CAD build for the part. Positions are in the model's coordinates, mm. Round coordinates to 2 decimals unless told otherwise and drop trailing zeros. Write each loop counter-clockwise with the first axis right and the second up, starting at its lowest first coordinate (ties: lowest second). Pieces come first, ordered by that corner, then holes. Notation, with made-up numbers: (49, 57.5) - (57, 57.5) arc R10 ccw to (57, 61.5) - close; hole circle Ø9 at (21.25, -9). An arc over 180 degrees is marked (long way). Answer in a Markdown table with one row per item.
```python
from build123d import *

# Parameters (mm, degrees)
SKETCH4_R           = 42.545
BOSS_EXTRUDE2_DEPTH = 0.254
SKETCH5_R           = 29.845
CUT_EXTRUDE5_DEPTH  = 1.254
SKETCH6_R           = 4.699
CUT_EXTRUDE6_DEPTH  = 1.254
SKETCH8_OUTSIDE_W   = 111.158
SKETCH8_OUTSIDE_H   = 111.158
CUT_EXTRUDE11_DEPTH = 1.254


with BuildPart() as part:
    # Sketch4 → Boss-Extrude2 (new body)
    with BuildSketch(Plane.XY):
        Circle(SKETCH4_R)
    extrude(amount=BOSS_EXTRUDE2_DEPTH)

    # Sketch5 → Cut-Extrude5 (cut, through all)
    with BuildSketch(Plane.XY.offset(0.254)):
        Circle(SKETCH5_R)
    extrude(amount=-CUT_EXTRUDE5_DEPTH, mode=Mode.SUBTRACT)

    # Sketch6 → Cut-Extrude6 (cut, through all)
    with BuildSketch(Plane.XY.offset(0.254)):
        with Locations((36.195, 0)):
            Circle(SKETCH6_R)
    extrude(amount=-CUT_EXTRUDE6_DEPTH, mode=Mode.SUBTRACT)

    # Sketch8 outside → Cut-Extrude11 (cut, through all)
    with BuildSketch(Plane.XY.offset(0.254)):
        Rectangle(SKETCH8_OUTSIDE_W, SKETCH8_OUTSIDE_H)
        with BuildLine():
            Line((28.034216891, -10.237514752), (39.774946424, -15.100684157))
            ThreePointArc((39.774946424, -15.100684157), (42.545, 0), (39.774946424, 15.100684157))
            Line((39.774946424, 15.100684157), (28.034216891, 10.237514752))
            ThreePointArc((28.034216891, 10.237514752), (29.845, 0), (28.034216891, -10.237514752))
        make_face(mode=Mode.SUBTRACT)
    extrude(amount=-CUT_EXTRUDE11_DEPTH, mode=Mode.SUBTRACT)


solid = part.part
```
Q1. Saw through at B-B on z = 0.1. List the corners of the cut face in (x, y) (3 decimals).
Computed:
| item | result |
|---|---|
| outline | (28.034, -10.238) - (39.775, -15.101) arc R42.545 ccw to (39.775, 15.101) - (28.034, 10.238) arc R29.845 cw to start; hole circle Ø9.398 at (36.195, 0) |
Q2. Saw through at C-C on x = 32. List the corners of the cut face in (y, z), then the cut area to 3 significant figures.
Computed:
| item | result |
|---|---|
| outline | (-11.88, 0) - (-2.12, 0) - (-2.12, 0.25) - (-11.88, 0.25) - close; (2.12, 0) - (11.88, 0) - (11.88, 0.25) - (2.12, 0.25) - close |
| area | 4.96 mm2 |
Q3. Drill centre lines: line 1 (Y direction, x = 32.5, z = 0.1); line 2 (Y direction, x = 36.25, z = 0.15); line 3 (X direction, y = -6, z = 0.2). Where is each one in solid material? Low to high.
Computed:
| item | result |
|---|---|
| line 1 | y = -12.09 to -2.9, 2.9 to 12.09 |
| line 2 | y = -13.64 to -4.7, 4.7 to 13.64 |
| line 3 | x = 29.24 to 42.12 |
Q4. Flat gauge pin, fed straight in: pin 1 (3 mm diameter, centred on x = 33, y = 1.5, fed in from -Z). Where does the tip first touch, or does it go through?
Computed:
| item | result |
|---|---|
| pin 1 | stops at z = 0 |
Q5. Saw through at D-D on y = -6. List the corners of the cut face in (x, z).
Computed:
| item | result |
|---|---|
| outline | (29.24, 0) - (42.12, 0) - (42.12, 0.25) - (29.24, 0.25) - close |
Q6. Saw through at A-A on y = 0. List the corners of the cut face in (x, z) (3 decimals), then the cut area to 3 significant figures.
Computed:
| item | result |
|---|---|
| outline | (29.845, 0) - (31.496, 0) - (31.496, 0.254) - (29.845, 0.254) - close; (40.894, 0) - (42.545, 0) - (42.545, 0.254) - (40.894, 0.254) - close |
| area | 0.839 mm2 |
